Design review of the part shown in the three views and the two pictorial views. Dimensions are in mm from the part's minimum x, y and z. A direction names the side the tool comes from. Give positions to 0.01 mm unless a question says otherwise; leave off trailing zeros. Loops run counter-clockwise (first coordinate to the right, second up) from the corner with the lowest first, then second, coordinate; pieces in that order, holes last. Notation, with made-up numbers: (86, 6.25) - (102, 6.25) arc R18 ccw to (102, 31.25) - close; hole circle Ø2 at (-2.5, 48). An arc over 180 degrees is marked (long way). Answer as a JSON object with one key per item and string values.
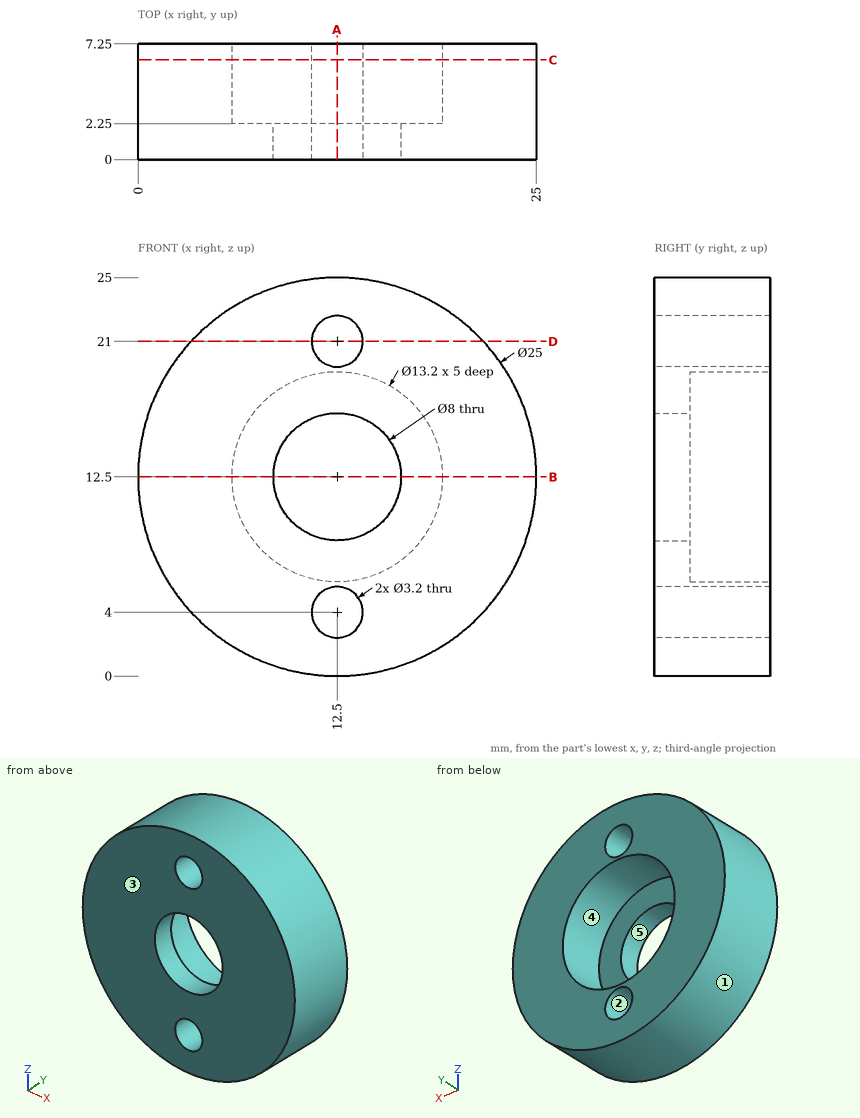
Q1. The part is to be moulded in two halves that separate along X. For the marked faces 1, 2 and 3, say which applies: +X half, -X half, draft (parallel to the pull), parting line (faces both ways), or undercut.
Results:
{"face 1": "parting line", "face 2": "undercut", "face 3": "draft"}
Q2. Consider section C-C, the plane y = 6.25. State the section outline as (x, z) points.
Results:
{"outline": "circle Ø25 at (12.5, 12.5); hole circle Ø13.2 at (12.5, 12.5); hole circle Ø3.2 at (12.5, 4); hole circle Ø3.2 at (12.5, 21)"}
Q3. To check wall thickness, follow probe 1 along Z at (x, y) = (12.5, 3.75); probe 2 along Z at (x, y) = (12.5, 2); probe 3 along X at (y, z) = (1.65, 12.5). State the ranges of each line that lie inside material, in increasing order. Write a range as [from, to].
Results:
{"probe 1": "z = [0, 2.4], [5.6, 5.9], [19.1, 19.4], [22.6, 25]", "probe 2": "z = [0, 2.4], [5.6, 8.5], [16.5, 19.4], [22.6, 25]", "probe 3": "x = [0, 8.5], [16.5, 25]"}
Q4. For the marked faces 4 and 5, list the 3-axis set-ups (+Z, -Z, +X, -X, +Y, -Y) from which the entire face can be reached by the end or side of a thin tool; tool diameter is ignored.
Results:
{"face 4": "+Y", "face 5": "+Y, -Y"}
Q5. Consider section A-A, the plane x = 12.5. State the section outline as (y, z) points.
Results:
{"outline": "(0, 0) - (7.25, 0) - (7.25, 2.4) - (0, 2.4) - close; (0, 5.6) - (7.25, 5.6) - (7.25, 5.9) - (2.25, 5.9) - (2.25, 8.5) - (0, 8.5) - close; (0, 16.5) - (2.25, 16.5) - (2.25, 19.1) - (7.25, 19.1) - (7.25, 19.4) - (0, 19.4) - close; (0, 22.6) - (7.25, 22.6) - (7.25, 25) - (0, 25) - close"}
Q6. Consider section D-D, the plane z = 21. State the section outline as (x, y) points, plus the area to 3 significant figures.
Results:
{"outline": "(3.33, 0) - (10.9, 0) - (10.9, 7.25) - (3.33, 7.25) - close; (14.1, 0) - (21.67, 0) - (21.67, 7.25) - (14.1, 7.25) - close", "area": "110 mm^2"}
Q7. Consider section B-B, the plane z = 12.5. State the section outline as (x, y) points.
Results:
{"outline": "(0, 0) - (8.5, 0) - (8.5, 2.25) - (5.9, 2.25) - (5.9, 7.25) - (0, 7.25) - close; (16.5, 0) - (25, 0) - (25, 7.25) - (19.1, 7.25) - (19.1, 2.25) - (16.5, 2.25) - close"}
Q8. Clearance check with flat-ended pins moving along their axes: pin 1 Ø1 at (x, z) = (13.5, 16) entering from +Y; pin 2 Ø3 at (x, z) = (11.5, 11.5) entering from +Y; pin 3 Ø1.5 at (y, z) = (6.5, 21) entering from +X; pin 4 Ø1 at (x, y) = (20, 2) entering from +Z. State where each tip first meets the part, or that it passes through.
Results:
{"pin 1": "stops at y = 2.25", "pin 2": "passes through", "pin 3": "stops at x = 22.31", "pin 4": "stops at z = 22.86"}
